Check sheet for the modelled part. Datum: model origin and axes. Units: mm. Face numbers are marked on the shaded views. Give positions to 0.01 mm unless a question says otherwise; leave off trailing zeros. Order: outer loops, then holes, each group sorted by start corner. A loop starts at its lowest first (then second) coordinate and runs counter-clockwise, first axis right, second up. Notation, with made-up numbers: M 82,42 L 111,42 A18 cw 111,76 Z; hole C 0,79.5 d10. An arc over 180 degrees is marked long. Return JSON: item names as keys, results as strings. Group by question number.
from build123d import *

# Parameters (mm, degrees)
EXTRUDE_1_DEPTH = 3
SKETCH_3_R      = 30
SKETCH_3_R_2    = 22.5
EXTRUDE_2_DEPTH = 1
SKETCH_4_R      = 25
SKETCH_4_R_2    = 22.5
EXTRUDE_3_DEPTH = 5


with BuildPart() as part:
    # 草图2 → 凸台-拉伸1 (new body)
    with BuildSketch(Plane.XY):
        with BuildLine():
            ThreePointArc((-116.606649797, -63.783530386), (-107.819853233, -84.996733821), (-86.606649797, -93.783530386))
            ThreePointArc((-86.606649797, -93.783530386), (-65.393446361, -84.996733821), (-56.606649797, -63.783530386))
            ThreePointArc((-56.606649797, -63.783530386), (-65.393446361, -42.57032695), (-86.606649797, -33.783530386))
            ThreePointArc((-86.606649797, -33.783530386), (-107.819853233, -42.57032695), (-116.606649797, -63.783530386))
        make_face()
        with BuildLine():
            ThreePointArc((-106.640989146, -48.829425703), (-102.516552374, -47.873627809), (-101.56075448, -43.749191037))
            ThreePointArc((-101.56075448, -43.749191037), (-86.606649797, -38.783530386), (-71.652545115, -43.749191037))
            ThreePointArc((-71.652545115, -43.749191037), (-70.69674722, -47.873627809), (-66.572310448, -48.829425703))
            ThreePointArc((-66.572310448, -48.829425703), (-61.606649797, -63.783530386), (-66.572310448, -78.737635068))
            ThreePointArc((-66.572310448, -78.737635068), (-70.69674722, -79.693432962), (-71.652545115, -83.817869734))
            ThreePointArc((-71.652545115, -83.817869734), (-86.606649797, -88.783530386), (-101.56075448, -83.817869734))
            ThreePointArc((-101.56075448, -83.817869734), (-102.516552374, -79.693432962), (-106.640989146, -78.737635068))
            ThreePointArc((-106.640989146, -78.737635068), (-111.606649797, -63.783530386), (-106.640989146, -48.829425703))
        make_face(mode=Mode.SUBTRACT)
    extrude(amount=EXTRUDE_1_DEPTH)

    # 草图3 → 凸台-拉伸2 (add)
    with BuildSketch(Plane.XY.offset(3)):
        with Locations((-86.606649797, -63.783530386)):
            Circle(SKETCH_3_R)
        with Locations(Location((-86.606649797, -63.783530386, 0), (0, 0, 135))):
            Circle(SKETCH_3_R_2, mode=Mode.SUBTRACT)
    extrude(amount=EXTRUDE_2_DEPTH)

    # 草图4 → 凸台-拉伸3 (add)
    with BuildSketch(Plane.XY.offset(4)):
        with Locations((-86.606649797, -63.783530386)):
            Circle(SKETCH_4_R)
        with Locations(Location((-86.606649797, -63.783530386, 0), (0, 0, 135))):
            Circle(SKETCH_4_R_2, mode=Mode.SUBTRACT)
    extrude(amount=EXTRUDE_3_DEPTH)


solid = part.part
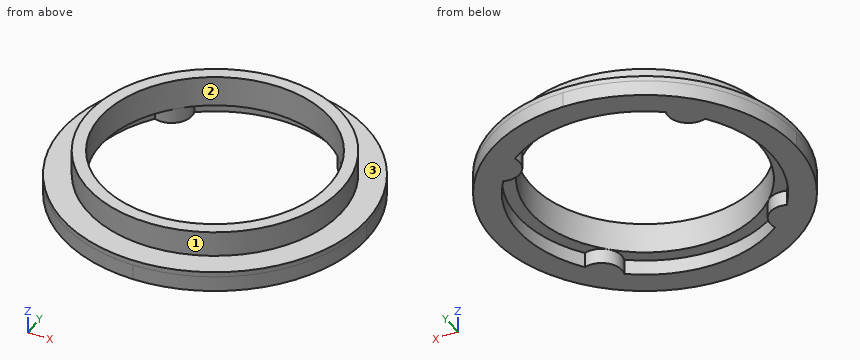
1) Depth check by flat-ended pin: P1, Ø1, axis at y = -84, z = 2.5, coming from the +X side; P2, Ø3, axis at y = -78.5, z = 1.5, coming from the -X side; P3, Ø1, axis at y = -54, z = 2.5, coming from the -X side; P4, Ø4.5, axis at x = -68, y = -62.5, coming from the -Z side. Enter the tip coordinate at first touch or a pass-through.
2) Sectioned sample at C-C on x = -96. Record the boundary of the cut face in (y, z), then the cut area to 3 significant figures.
3) Release check for a two-part mould opening along Y. For the marked faces 1, 2 and 3 record: released by +Y, released by -Y, zero draft, split by the parting line, or undercut.
4) Sectioned sample at A-A on z = 1.5. Record the boundary of the cut face in (x, y).
5) Sectioned sample at B-B on y = -51. Record the boundary of the cut face in (x, z).
6) Sectioned sample at D-D on z = 6.5. Record the boundary of the cut face in (x, y), then the cut area to 3 significant figures.
7) Material ranges on line 1 along Y through (x, z) = (-97.5, 1.75); line 2 along Y through (x, z) = (-87.5, 6); line 3 along X through (y, z) = (-82.5, 2.75), recorded low to high.
Reply:
{
 "1": {"P1": "x = -64", "P2": "x = -113.54", "P3": "x = -115.13", "P4": "through"},
 "2": {"outline": "M -92.28,0 L -86.95,0 L -86.95,3 L -84.23,3 L -84.23,9 L -86.95,9 L -86.95,4 L -92.28,4 Z; M -43.34,3 L -40.62,3 L -40.62,0 L -35.29,0 L -35.29,4 L -40.62,4 L -40.62,9 L -43.34,9 Z", "area": "75.3 mm^2"},
 "3": {"face 1": "split by the parting line", "face 2": "undercut", "face 3": "zero draft"},
 "4": {"outline": "C -86.61,-63.78 d60; hole M -106.64,-78.74 A4 cw -101.56,-83.82 A25 ccw -71.65,-83.82 A4 cw -66.57,-78.74 A25 ccw -66.57,-48.83 A4 cw -71.65,-43.75 A25 ccw -101.56,-43.75 A4 cw -106.64,-48.83 A25 ccw Z"},
 "5": {"outline": "M -113.75,0 L -108.09,0 L -108.09,3 L -105.12,3 L -105.12,9 L -108.09,9 L -108.09,4 L -113.75,4 Z; M -68.09,3 L -65.12,3 L -65.12,0 L -59.47,0 L -59.47,4 L -65.12,4 L -65.12,9 L -68.09,9 Z"},
 "6": {"outline": "C -86.61,-63.78 d50; hole C -86.61,-63.78 d45", "area": "373 mm^2"},
 "7": {"line 1": "-91.74 to -86.29, -41.28 to -35.83", "line 2": "-88.77 to -86.27, -41.3 to -38.8", "line 3": "-110.05 to -101.35, -71.87 to -63.16"}
}
